```python
from build123d import *

# Parameters (mm, degrees)
SKETCH_1_W          = 42.3
SKETCH_1_H          = 42.3
EXTRUDE_1_DEPTH     = 38
SKETCH_3_R          = 1.5
CUT_EXTRUDE_1_DEPTH = 4.5
SKETCH_4_R          = 8
SKETCH_4_R_2        = 2.5
EXTRUDE_2_DEPTH     = 2
SKETCH_5_R          = 2.25
EXTRUDE_3_DEPTH     = 24
CUT_EXTRUDE_2_DEPTH = 24
FILLET_1_R          = 1
CUT_EXTRUDE_START   = -8
SKETCH_10_W         = 42.3
SKETCH_10_H         = 42.3
SKETCH_10_W_2       = 40.3
SKETCH_10_H_2       = 40.3
CUT_EXTRUDE_4_DEPTH = 22
FILLET_2_R          = 1
SKETCH_11_W         = 16.2
SKETCH_11_H         = 9.4
EXTRUDE_4_DEPTH     = 4


with BuildPart() as part:
    # 草图1 → 凸台-拉伸1 (new body)
    with BuildSketch(Plane.XY):
        with Locations((21.15, 21.15)):
            Rectangle(SKETCH_1_W, SKETCH_1_H)
    extrude(amount=EXTRUDE_1_DEPTH)

    # 草图3 → 切除-拉伸1 (cut)
    with BuildSketch(Plane.XY.offset(38)):
        with Locations((5.65, 36.65)):
            Circle(SKETCH_3_R)
        with Locations((36.65, 36.65)):
            Circle(SKETCH_3_R)
        with Locations(Location((36.65, 5.65, 0), (0, 0, 180))):
            Circle(SKETCH_3_R)
        with Locations(Location((5.65, 5.65, 0), (0, 0, 180))):
            Circle(SKETCH_3_R)
    extrude(amount=-CUT_EXTRUDE_1_DEPTH, mode=Mode.SUBTRACT)

    # 草图4 → 凸台-拉伸2 (add)
    with BuildSketch(Plane.XY.offset(38)):
        with Locations((21.15, 21.15)):
            Circle(SKETCH_4_R)
        with Locations((21.15, 21.15)):
            Circle(SKETCH_4_R_2, mode=Mode.SUBTRACT)
    extrude(amount=EXTRUDE_2_DEPTH)

    # 草图5 → 凸台-拉伸3 (add)
    with BuildSketch(Plane.XY.offset(38)):
        with Locations(Location((21.15, 21.15, 0), (0, 0, 180))):
            Circle(SKETCH_5_R)
    extrude(amount=EXTRUDE_3_DEPTH)

    # 草图6 → 切除-拉伸2 (cut)
    with BuildSketch(Plane(origin=(0, 0, 0), x_dir=(0, 0, -1), z_dir=(1, 0, 0))):
        Polygon((-62, 22.9), (-45, 22.9), (-44, 23.4), (-62, 23.4), align=None)
    extrude(amount=CUT_EXTRUDE_2_DEPTH, mode=Mode.SUBTRACT)

    # 草图9 → 切除-旋转1 (revolve, cut)
    with BuildSketch(Plane(origin=(0, 21.15, 0), x_dir=(1, 0, 0), z_dir=(0, 1, 0)), mode=Mode.PRIVATE) as cut_revolve_1_sk:
        Polygon((23.4, -61.739352103), (22.6, -62.201232319), (23.4, -62.201232319), align=None)
    revolve(cut_revolve_1_sk.sketch.rotate(Axis((21.15, 21.15, 62), (0, 0, -1)), 180), axis=Axis((21.15, 21.15, 62), (0, 0, -1)), mode=Mode.SUBTRACT)

    # 圆角1
    fillet_1_edges = [part.edges().sort_by_distance(p)[0] for p in [
        (42.3, 21.15, 38),
        (21.15, 42.3, 38),
        (0, 21.15, 38),
        (21.15, 42.3, 0),
        (42.3, 21.15, 0),
        (21.15, 0, 0),
        (0, 21.15, 0),
        (0, 42.3, 19),
        (42.3, 42.3, 19),
        (42.3, 0, 19),
        (0, 0, 19),
        (21.15, 0, 38),
    ]]
    fillet(fillet_1_edges, radius=FILLET_1_R)

    # 草图10 → 切除-拉伸4 (cut)
    with BuildSketch(Plane.XY.offset(38).offset(CUT_EXTRUDE_START)):
        with Locations((21.15, 21.15)):
            Rectangle(SKETCH_10_W, SKETCH_10_H)
        with Locations((21.15, 21.15)):
            Rectangle(SKETCH_10_W_2, SKETCH_10_H_2, mode=Mode.SUBTRACT)
    extrude(amount=-CUT_EXTRUDE_4_DEPTH, mode=Mode.SUBTRACT)

    # 圆角2
    fillet_2_edges = [part.edges().sort_by_distance(p)[0] for p in [
        (0.292893219, 0.292893219, 30),
        (0.292893219, 0.292893219, 8),
        (42.3, 21.15, 8),
        (21.15, 42.3, 8),
        (0, 21.15, 8),
        (21.15, 0, 8),
        (42.007106781, 42.007106781, 30),
        (42.007106781, 0.292893219, 30),
        (0.292893219, 42.007106781, 30),
        (42.007106781, 42.007106781, 8),
        (42.007106781, 0.292893219, 8),
        (0.292893219, 42.007106781, 8),
        (21.15, 42.3, 30),
        (0, 21.15, 30),
        (21.15, 0, 30),
        (42.3, 21.15, 30),
    ]]
    fillet(fillet_2_edges, radius=FILLET_2_R - 0.0001)  # a hair under: the kernel refuses the full size

    # 草图11 → 凸台-拉伸4 (add)
    with BuildSketch(Plane(origin=(0, 42.3, 0), x_dir=(1, 0, 0), z_dir=(0, 1, 0))):
        with Locations((21.15, -4.7)):
            Rectangle(SKETCH_11_W, SKETCH_11_H)
    extrude(amount=EXTRUDE_4_DEPTH)


solid = part.part
```
Can you work these out from the model? Positions are in its coordinate system, mm. A direction names the side the tool comes from. Coordinates: 2 decimals unless noted, no trailing zeros. Loops run counter-clockwise (first coordinate to the right, second up) from the corner with the lowest first, then second, coordinate; pieces in that order, holes last. Notation, with made-up numbers: M -23.75,1.25 L -4.75,1.25 A32 cw -4.75,37.25 Z; hole C 37.5,-25.75 d2. An arc over 180 degrees is marked long. Put each result on its own line as item: value. Start each with the question number.
(1) Imagine slicing it at C-C on z = 6. List the corners of the cut face in (x, y) for me, and give its area (3 significant figures).
(2) I need wall thicknesses on probe 1 along Y at (x, z) = (5.65, 35.95); probe 2 along X at (y, z) = (21, 39) (1 decimal). Which ranges of each line are inside material? Lowest first, please.
(3) We'd pull the mould along X, two halves only. Please class faces 6 (the face through (6, 37, 33.5)), 7 (the face through (29.25, 44, 5)), 8 (the face through (37, 6, 33.5)), 9 (the face through (35, 42.3, 4)): +X half, -X half, draft (parallel to the pull), parting line (faces both ways), or undercut.
(4) Which directions (+Z, -Z, +X, -X, +Y, -Y) give clear straight access to the entire face, cutting with the end or side of a thin tool? Please do faces 1 (the face through (21, 1, 19)), 2 (the face through (21, 21, 62)), 3 (the face through (21, 44, 9.4)), 4 (the face through (13.05, 44, 5)), 5 (the face through (6, 6, 33.5)).
(5) Will these pins go through, and if not, where does the flat tip stop? pin 1 Ø5 at (y, z) = (38.5, 15) entering from -X; pin 2 Ø2 at (y, z) = (37, 22.5) entering from +X; pin 3 Ø2 at (x, y) = (32.5, 25) entering from +Z; pin 4 Ø20 at (x, y) = (28, 28.5) entering from +Z.
Worked answers:
1. outline: M 0,1 A1 ccw 1,0 L 41.3,0 A1 ccw 42.3,1 L 42.3,41.3 A1 ccw 41.3,42.3 L 29.25,42.3 L 29.25,46.3 L 13.05,46.3 L 13.05,42.3 L 1,42.3 A1 ccw 0,41.3 Z
1. area: 1,850 mm2
2. probe 1: y = 0 to 4.15, 7.15 to 35.15, 38.15 to 42.3
2. probe 2: x = 13.2 to 18.7, 18.9 to 23.4, 23.6 to 29.1
3. face 6: undercut
3. face 7: +X half
3. face 8: undercut
3. face 9: draft
4. face 1: +X, -X, -Y
4. face 2: +Z, +X, -X, +Y, -Y
4. face 3: +Z, +X, -X, +Y
4. face 4: +Z, -Z, -X, +Y
4. face 5: +Z
5. pin 1: stops at x = 1
5. pin 2: stops at x = 41.3
5. pin 3: stops at z = 38
5. pin 4: stops at z = 62
